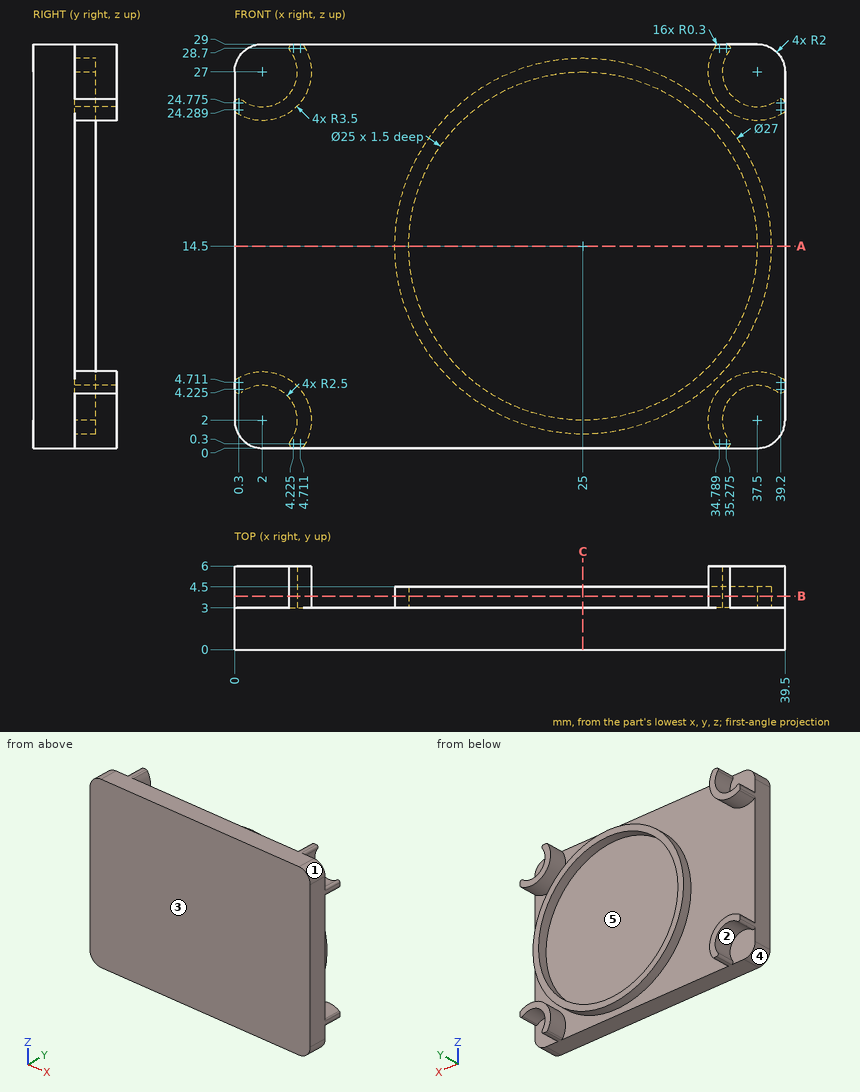
Check sheet for the drawn part. Datum: minimum x, y, z corner. Units: mm. A direction names the side the tool comes from. Coordinates: 2 decimals unless noted, no trailing zeros. Loops run counter-clockwise (first coordinate to the right, second up) from the corner with the lowest first, then second, coordinate; pieces in that order, holes last. Notation, with made-up numbers: (-19, 7) -> (35, 7) arc R25 cw to (35, 46) -> close; hole circle Ø2 at (56, 39.25). An arc over 180 degrees is marked (long way). Answer as a JSON object with one key per item and string values. Group by question number.
Item 1: Tool access check on the marked faces 1 and 2. Record the directions out of +Z, -Z, +X, -X, +Y, -Y that give a thin tool (end or side, any length) a straight path to the whole face; none if there is none.
Item 2: Sectioned sample at A-A on z = 14.5. Record the boundary of the cut face in (x, y).
Item 3: Mould release check, pull along Z, two halves, no side actions. Record for the marked faces 3, 4 and 5: +Z half, -Z half, draft (parallel to the pull), parting line (faces both ways), or undercut.
Item 4: Sectioned sample at B-B on y = 3.85. State how many separate pieces and enclosed holes the cut face has, plus the area to 3 significant figures.
Item 5: Sectioned sample at C-C on x = 25. Record the boundary of the cut face in (y, z).
Item 6: Depth check by flat-ended pin: pin 1 (1.4 mm diameter, centred on x = 2, z = 26.5, fed in from +Y); pin 2 (1.5 mm diameter, centred on x = 19, y = 4, fed in from -Z). Enter the tip coordinate at first touch or a pass-through.
Item 7: Scan lines: probe 1 along X at (y, z) = (3.75, 14.5); probe 2 along Y at (x, z) = (10, 19); probe 3 along Y at (x, z) = (26, 1.75). Record each from-to range of solid material in increasing order.
Evaluation:
{
 "1": {"face 1": "+Z, +X, +Y, -Y", "face 2": "+Y"},
 "2": {"outline": "(0, 0) -> (39.5, 0) -> (39.5, 3) -> (38.5, 3) -> (38.5, 4.5) -> (37.5, 4.5) -> (37.5, 3) -> (12.5, 3) -> (12.5, 4.5) -> (11.5, 4.5) -> (11.5, 3) -> (0, 3) -> close"},
 "3": {"face 3": "draft", "face 4": "-Z half", "face 5": "undercut"},
 "4": {"separate pieces": "5", "enclosed holes": "1", "area": "117 mm²"},
 "5": {"outline": "(0, 0) -> (3, 0) -> (3, 1) -> (4.5, 1) -> (4.5, 2) -> (3, 2) -> (3, 27) -> (4.5, 27) -> (4.5, 28) -> (3, 28) -> (3, 29) -> (0, 29) -> close"},
 "6": {"pin 1": "stops at y = 3", "pin 2": "stops at z = 2.06"},
 "7": {"probe 1": "x = 11.5 to 12.5, 37.5 to 38.5", "probe 2": "y = 0 to 3", "probe 3": "y = 0 to 4.5"}
}
